For this review, take the finished solid that the model builds, in its own axes (mm). Face numbers are marked on the shaded views. A direction names the side the tool comes from. Give positions to 0.01 mm unless a question says otherwise; leave off trailing zeros. Loops run counter-clockwise (first coordinate to the right, second up) from the corner with the lowest first, then second, coordinate; pieces in that order, holes last. Notation, with made-up numbers: (71.25, -16.75) - (93.25, -16.75) arc R24 ccw to (93.25, -1.75) - close; hole circle Ø4 at (-17, 49). An arc over 180 degrees is marked (long way). Answer in a Markdown table with one row per item.
```python
from build123d import *

# Parameters (mm, degrees)
BOSS_EXTRUDE1_DEPTH                                 = 80
CBORE_FOR_M6_HEX_SOCKET_HEAD_CAP_SCREW1_D           = 6.6
CBORE_FOR_M6_HEX_SOCKET_HEAD_CAP_SCREW1_CBORE_D     = 11
CBORE_FOR_M6_HEX_SOCKET_HEAD_CAP_SCREW1_CBORE_DEPTH = 6.4
FILLET1_R                                           = 0.5
FILLET2_R                                           = 1
CHAMFER1_SIZE                                       = 0.5
CHAMFER2_SIZE                                       = 0.5


with BuildPart() as part:
    # Sketch2 → Boss-Extrude1 (new body)
    with BuildSketch(Plane(origin=(0, 0, 0), x_dir=(0, 0, -1), z_dir=(1, 0, 0))):
        Polygon((0, 0), (0, 53), (-10, 43), (-10, 10), align=None)
    extrude(amount=BOSS_EXTRUDE1_DEPTH)

    # CBORE for M6 Hex Socket Head Cap Screw1 (through all)
    with Locations(Plane(origin=(0, 0, 0), x_dir=(-1, 0, 0), z_dir=(0, 0, -1))):
        with Locations((-70, 17.5), (-10, 17.5)):
            CounterBoreHole(CBORE_FOR_M6_HEX_SOCKET_HEAD_CAP_SCREW1_D / 2, CBORE_FOR_M6_HEX_SOCKET_HEAD_CAP_SCREW1_CBORE_D / 2, CBORE_FOR_M6_HEX_SOCKET_HEAD_CAP_SCREW1_CBORE_DEPTH)

    # Fillet1
    fillet1_edges = [part.edges().sort_by_distance(p)[0] for p in [
        (40, 53, 0),
        (40, 0, 0),
    ]]
    fillet(fillet1_edges, radius=FILLET1_R)

    # Fillet2
    fillet2_edges = [part.edges().sort_by_distance(p)[0] for p in [
        (40, 10, 10),
        (40, 43, 10),
    ]]
    fillet(fillet2_edges, radius=FILLET2_R)

    # Chamfer1
    chamfer1_edges = [part.edges().sort_by_distance(p)[0] for p in [
        (6.7, 17.5, 10),
        (66.7, 17.5, 10),
        (0, 47.719669914, 5.280330086),
        (80, 47.719669914, 5.280330086),
        (0, 26.5, 0),
        (0, 0.745167015, 0.308658284),
        (0, 52.254832985, 0.308658284),
        (80, 26.5, 0),
        (80, 0.745167015, 0.308658284),
        (80, 52.254832985, 0.308658284),
        (0, 26.5, 10),
        (80, 26.5, 10),
        (0, 5.280330086, 5.280330086),
        (0, 10.03153013, 9.923879533),
        (0, 42.96846987, 9.923879533),
        (80, 5.280330086, 5.280330086),
        (80, 10.03153013, 9.923879533),
        (80, 42.96846987, 9.923879533),
    ]]
    chamfer(chamfer1_edges, length=CHAMFER1_SIZE)

    # Chamfer2
    chamfer2_edges = [part.edges().sort_by_distance(p)[0] for p in [
        (15.5, 17.5, 0),
        (75.5, 17.5, 0),
    ]]
    chamfer(chamfer2_edges, length=CHAMFER2_SIZE)


solid = part.part
```
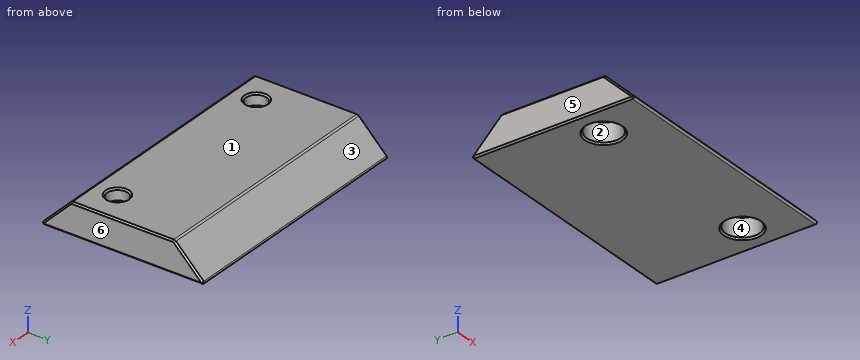
1. We need section A-A, the plane x = 10. Give the boundary of the cut face in (y, z).
Values:
| item | result |
|---|---|
| outline | (0.85, 0.85) arc R0.5 ccw to (1.21, 0) - (11.5, 0) - (12, 0.5) - (12, 6.4) - (14.2, 6.4) - (14.2, 9.5) - (13.7, 10) - (10.41, 10) arc R1 ccw to (9.71, 9.71) - close; (20.8, 6.4) - (23, 6.4) - (23, 0.5) - (23.5, 0) - (51.79, 0) arc R0.5 ccw to (52.15, 0.85) - (43.29, 9.71) arc R1 ccw to (42.59, 10) - (21.3, 10) - (20.8, 9.5) - close |
2. We need section D-D, the plane y = 48. Give the boundary of the cut face in (x, z), and give its area (3 significant figures).
Values:
| item | result |
|---|---|
| outline | (0, 0.5) - (0.5, 0) - (79.5, 0) - (80, 0.5) - (80, 4.29) - (79.5, 5) - (0.5, 5) - (0, 4.29) - close |
| area | 399 mm^2 |
3. Clearance check with flat-ended pins moving along their axes: pin 1 (4 mm diameter, centred on x = 54.5, z = 8, fed in from +Y); pin 2 (12 mm diameter, centred on x = 70.5, y = 16, fed in from -Z); pin 3 (1 mm diameter, centred on x = 51, z = 8, fed in from +Y); pin 4 (6 mm diameter, centred on x = 28.5, z = 4.5, fed in from +Y). State where each tip first meets the part, or that it passes through.
Values:
| item | result |
|---|---|
| pin 1 | stops at y = 47 |
| pin 2 | stops at z = 0 |
| pin 3 | stops at y = 45.5 |
| pin 4 | stops at y = 51.5 |
4. We need section B-B, the plane y = 17.5. Count the separate pieces of the cut face and the enclosed holes in it, and give its area (3 significant figures).
Values:
| item | result |
|---|---|
| separate pieces | 3 |
| enclosed holes | 0 |
| area | 610 mm^2 |
5. Mouldability with a two-part tool opening along X and no side actions: class the marked faces 3, 4, 5 and 6 as released by +X, released by -X, zero draft, split by the parting line, or undercut.
Values:
| item | result |
|---|---|
| face 3 | zero draft |
| face 4 | undercut |
| face 5 | released by -X |
| face 6 | released by +X |
6. We need section C-C, the plane z = 5.5. Give the boundary of the cut face in (x, y), and give its area (3 significant figures).
Values:
| item | result |
|---|---|
| outline | (0, 6.21) - (0.5, 5.5) - (79.5, 5.5) - (80, 6.21) - (80, 46.79) - (79.5, 47.5) - (0.5, 47.5) - (0, 46.79) - close; hole circle Ø11 at (10, 17.5); hole circle Ø11 at (70, 17.5) |
| area | 3,170 mm^2 |
7. Wall thickness on line 1 (X direction, y = 21, z = 2); line 2 (Y direction, x = 10, z = 4.3); line 3 (Y direction, x = 70, z = 2.6): over which ranges is each line inside the solid? List them lowest first. Write a range as [from, to].
Values:
| item | result |
|---|---|
| line 1 | x = [0, 5.76], [14.24, 65.76], [74.24, 80] |
| line 2 | y = [4.3, 12], [23, 48.7] |
| line 3 | y = [2.6, 12], [23, 50.4] |
8. For the marked faces 1 and 2, list the 3-axis set-ups (+Z, -Z, +X, -X, +Y, -Y) from which the entire face can be reached by the end or side of a thin tool; tool diameter is ignored.
Values:
| item | result |
|---|---|
| face 1 | +Z, +X, -X, +Y, -Y |
| face 2 | -Z |
